from build123d import *

# Parameters (mm, degrees)
SKETCH4_R           = 50
BOSS_EXTRUDE3_DEPTH = 45.1
SKETCH16_R          = 4.5
BOSS_EXTRUDE5_DEPTH = 15
SKETCH5_W           = 42.3
SKETCH5_H           = 42.3
CUT_EXTRUDE1_DEPTH  = 39.8
SKETCH7_W           = 16.113230219
SKETCH7_H           = 35.470323835
CUT_EXTRUDE3_DEPTH  = 11
SKETCH8_R           = 11.15
SKETCH8_R_2         = 1.65
CUT_EXTRUDE4_DEPTH  = 5.3
SKETCH9_R           = 2.9
CUT_EXTRUDE5_DEPTH  = 3.2
BOSS_EXTRUDE4_DEPTH = 15


with BuildPart() as part:
    # Sketch4 → Boss-Extrude3 (new body)
    with BuildSketch(Plane(origin=(0, 39.8, 0), x_dir=(1, 0, 0), z_dir=(0, 1, 0))):
        with Locations(Location((-8.113230219, -47.62731131, 0), (0, 0, 270))):
            Circle(SKETCH4_R)
    extrude(amount=-BOSS_EXTRUDE3_DEPTH)

    # Sketch16 → Boss-Extrude5 (add)
    with BuildSketch(Plane.XZ.offset(5.3)):
        with Locations(Location((-8.113230219, 21.53731131, 0), (0, 0, 90))):
            Circle(SKETCH16_R)
        with Locations(Location((17.976769781, 47.62731131, 0), (0, 0, 90))):
            Circle(SKETCH16_R)
        with Locations(Location((-8.113230219, 73.71731131, 0), (0, 0, 90))):
            Circle(SKETCH16_R)
        with Locations(Location((-34.203230219, 47.62731131, 0), (0, 0, 90))):
            Circle(SKETCH16_R)
        with Locations(Location((-32.86196756, 22.878573969, 0), (0, 0, 90))):
            Circle(SKETCH16_R)
        with Locations(Location((16.635507123, 22.878573969, 0), (0, 0, 90))):
            Circle(SKETCH16_R)
        with Locations(Location((16.635507123, 72.376048652, 0), (0, 0, 90))):
            Circle(SKETCH16_R)
        with Locations(Location((-32.86196756, 72.376048652, 0), (0, 0, 90))):
            Circle(SKETCH16_R)
    extrude(amount=BOSS_EXTRUDE5_DEPTH)

    # Sketch5 → Cut-Extrude1 (cut)
    with BuildSketch(Plane(origin=(0, 39.8, 0), x_dir=(1, 0, 0), z_dir=(0, 1, 0))):
        with Locations((-8.113230219, -47.62731131)):
            Rectangle(SKETCH5_W, SKETCH5_H)
    extrude(amount=-CUT_EXTRUDE1_DEPTH, mode=Mode.SUBTRACT)

    # Sketch7 → Cut-Extrude3 (cut)
    with BuildSketch(Plane(origin=(0, 39.8, 0), x_dir=(1, 0, 0), z_dir=(0, 1, 0))):
        with Locations((-8.05661511, -86.512473228)):
            Rectangle(SKETCH7_W, SKETCH7_H)
    extrude(amount=-CUT_EXTRUDE3_DEPTH, mode=Mode.SUBTRACT)

    # Sketch8 → Cut-Extrude4 (cut)
    with BuildSketch(Plane(origin=(0, 0, 0), x_dir=(1, 0, 0), z_dir=(0, 1, 0))):
        with Locations(Location((-8.113230219, -47.62731131, 0), (0, 0, 270))):
            Circle(SKETCH8_R)
        with Locations(Location((7.386769781, -32.12731131, 0), (0, 0, 270))):
            Circle(SKETCH8_R_2)
        with Locations(Location((7.386769781, -63.12731131, 0), (0, 0, 270))):
            Circle(SKETCH8_R_2)
        with Locations(Location((-23.613230219, -63.12731131, 0), (0, 0, 270))):
            Circle(SKETCH8_R_2)
        with Locations(Location((-23.613230219, -32.12731131, 0), (0, 0, 270))):
            Circle(SKETCH8_R_2)
    extrude(amount=-CUT_EXTRUDE4_DEPTH, mode=Mode.SUBTRACT)

    # Sketch9 → Cut-Extrude5 (cut)
    with BuildSketch(Plane.XZ.offset(5.3)):
        with Locations(Location((-23.613230219, 32.12731131, 0), (0, 0, 270))):
            Circle(SKETCH9_R)
        with Locations(Location((-23.613230219, 63.12731131, 0), (0, 0, 270))):
            Circle(SKETCH9_R)
        with Locations(Location((7.386769781, 63.12731131, 0), (0, 0, 270))):
            Circle(SKETCH9_R)
        with Locations(Location((7.386769781, 32.12731131, 0), (0, 0, 270))):
            Circle(SKETCH9_R)
    extrude(amount=-CUT_EXTRUDE5_DEPTH, mode=Mode.SUBTRACT)

    # Sketch11 → Boss-Extrude4 (add)
    with BuildSketch(Plane(origin=(0, 39.8, 0), x_dir=(1, 0, 0), z_dir=(0, 1, 0))):
        with BuildLine():
            Line((-29.345351576, 192.94147664), (-28.113230219, -1.801554361))
            ThreePointArc((-28.113230219, -1.801554361), (-8.113230219, 2.37268869), (11.886769781, -1.801554361))
            Line((11.886769781, -1.801554361), (10.653047297, 193.194542854))
            ThreePointArc((10.653047297, 193.194542854), (9.166241961, 196.720740641), (5.621513459, 198.162808872))
            Line((5.621513459, 198.162808872), (-24.377085557, 197.973010478))
            ThreePointArc((-24.377085557, 197.973010478), (-27.903283344, 196.486205142), (-29.345351576, 192.94147664))
        make_face()
        with BuildLine():
            Line((232.962144958, -27.62731131), (37.712526731, -27.62731131))
            ThreePointArc((37.712526731, -27.62731131), (41.886769781, -47.62731131), (37.712526731, -67.62731131))
            Line((37.712526731, -67.62731131), (232.707755381, -68.991424164))
            ThreePointArc((232.707755381, -68.991424164), (236.253447378, -67.551726556), (237.742610291, -64.026523759))
            Line((237.742610291, -64.026523759), (237.962022615, -32.662288563))
            ThreePointArc((237.962022615, -32.662288563), (236.510023638, -29.104165434), (232.962144958, -27.62731131))
        make_face()
        with BuildLine():
            ThreePointArc((-54.659069334, -65.888879179), (-43.468569278, -82.98265037), (-26.374798087, -94.173150426))
            Line((-26.374798087, -94.173150426), (-66.449539667, -130.7123581))
            Line((-66.449539667, -130.7123581), (-91.198277008, -105.963620758))
            Line((-91.198277008, -105.963620758), (-54.659069334, -65.888879179))
        make_face()
    extrude(amount=-BOSS_EXTRUDE4_DEPTH)


solid = part.part
Verification items for the finished model (mm, model axes). A direction names the side the tool comes from. Coordinates: 2 decimals unless noted, no trailing zeros. Order: outer loops, then holes, each group sorted by start corner. A loop starts at its lowest first (then second) coordinate and runs counter-clockwise, first axis right, second up. Notation, with made-up numbers: M 72.5,79 L 81.5,79 A25 cw 81.5,97 Z; hole C 6.25,85.25 d11. An arc over 180 degrees is marked long. Write each question's results on one line, items separated by ' | '.
1) Access from +Z, -Z, +X, -X, +Y, -Y to the whole of each face (thin tool, end or side, straight path). Record for faces 5 (the face through (137, 32, 27.627)), 6 (the face through (-16.113, 34, 83)), 7 (the face through (-8, 20, 68.777)), 8 (the face through (-36.656, -12.695, 25.298)).
Solved:
face 5: -Z, +X, +Y, -Y | face 6: +Z, +Y | face 7: +Y | face 8: -Y
2) Gauge pin test, flat ends, axial feed: pin 1 Ø1.5 at (y, z) = (-4, 7.5) entering from +X; pin 2 Ø9.5 at (x, z) = (-23.61, 63.13) entering from +Y; pin 3 Ø12.5 at (x, z) = (-6, -112.5) entering from -Y. Record the tip position at first contact, or that the pin passes through.
Solved:
pin 1: stops at x = 22.7 | pin 2: stops at y = 0 | pin 3: stops at y = 24.8
3) Scan lines: line 1 along X through (y, z) = (20, 40); line 2 along Y through (x, z) = (13, 66.5); line 3 along X through (y, z) = (32.5, -182.5). Record each from-to range of solid material in increasing order. Write a range as [from, to].
Solved:
line 1: x = [-57.53, -29.26], [13.04, 41.3] | line 2: y = [-5.3, 0] | line 3: x = [-29.28, 10.72]
4) Section check D-D on z = -48. Record the cut outline in (x, y), plus the area to 3 significant figures.
Solved:
outline: M -28.43,24.8 L 11.57,24.8 L 11.57,39.8 L -28.43,39.8 Z | area: 600 mm²
5) Release check for a two-part mould opening along Z. For faces 1 (the face through (-8.31, -12.7, 69.22)), 2 (the face through (-33, -20.3, 72)), 3 (the face through (-8, 20, 26.477)), 4 (the face through (-46.132, 32.405, 112.187)) record: pulls with the +Z half, pulls with the -Z half, needs draft (parallel to the pull), parting line crosses it, or undercut.
Solved:
face 1: undercut | face 2: needs draft | face 3: undercut | face 4: pulls with the +Z half
6) Section check B-B on x = -44. Record the cut outline in (y, z).
Solved:
outline: M -5.3,12.81 L 39.8,12.81 L 39.8,110.24 L 24.8,110.24 L 24.8,82.44 L -5.3,82.44 Z
7) Section check C-C on y = 8.5. Record the cut outline in (x, z), plus the area to 3 significant figures.
Solved:
outline: C -8.11,47.63 d100; hole M -29.26,26.48 L 13.04,26.48 L 13.04,68.78 L -29.26,68.78 Z | area: 6,060 mm²
8) Section check A-A on y = 33.5. Record the cut outline in (x, z), plus the area to 3 significant figures.
Solved:
outline: M -91.2,105.96 L -54.66,65.89 A50 ccw -28.11,1.8 L -29.35,-192.94 A5 ccw -24.38,-197.97 L 5.62,-198.16 A5 ccw 10.65,-193.19 L 11.89,1.8 A50 ccw 37.71,27.63 L 232.96,27.63 A5 ccw 237.96,32.66 L 237.74,64.03 A5 ccw 232.71,68.99 L 37.71,67.63 A50 ccw 0,96.96 L 0,68.78 L 13.04,68.78 L 13.04,26.48 L -29.26,26.48 L -29.26,68.78 L -16.11,68.78 L -16.11,96.98 A50 ccw -26.37,94.17 L -66.45,130.71 Z | area: 23,400 mm²
